from build123d import *

# Parameters (mm, degrees)
EXTRUDE_590_DEPTH   = 27.6
EXTRUDE_638_DEPTH   = 9.5
FILLET_1_R          = 3
HOLE_WIZARD_M5_1_D  = 5.3
CUT_EXTRUDE_1_DEPTH = 5
CUT_EXTRUDE_2_DEPTH = 0.1


with BuildPart() as part:
    # 草图1 → Extrude 590 (new body)
    with BuildSketch(Plane(origin=(0, 0, 0), x_dir=(1, 0, 0), z_dir=(0, 1, 0))):
        with BuildLine():
            Line((4.608867317, -165), (-4.608867317, -165))
            Line((-4.608867317, -165), (-5.444719551, -194.923972433))
            ThreePointArc((-5.444719551, -194.923972433), (0, -195), (5.444719551, -194.923972433))
            Line((5.444719551, -194.923972433), (4.608867317, -165))
        make_face()
    extrude(amount=EXTRUDE_590_DEPTH)

    # 草图1<3> → Extrude 638 (add)
    with BuildSketch(Plane(origin=(0, 0, 0), x_dir=(1, 0, 0), z_dir=(0, 1, 0))):
        with BuildLine():
            ThreePointArc((5.444719551, -194.923972433), (0, -195), (-5.444719551, -194.923972433))
            Line((-5.444719551, -194.923972433), (-5.584327745, -199.922023008))
            ThreePointArc((-5.584327745, -199.922023008), (0, -200), (5.584327745, -199.922023008))
            Line((5.584327745, -199.922023008), (5.444719551, -194.923972433))
        make_face()
    extrude(amount=EXTRUDE_638_DEPTH)

    # 圆角1
    fillet_1_edges = [part.edges().sort_by_distance(p)[0] for p in [
        (0, 0, 165),
        (-4.608867317, 13.8, 165),
        (4.608867317, 13.8, 165),
    ]]
    fillet(fillet_1_edges, radius=FILLET_1_R)

    # M5 间隙孔1 (through all)
    with Locations(Plane(origin=(0, 27.6, 0), x_dir=(1, 0, 0), z_dir=(0, 1, 0))):
        with Locations((0, -187), (0, -175)):
            Hole(HOLE_WIZARD_M5_1_D / 2)

    # 草图6 → 切除-拉伸1 (cut)
    with BuildSketch(Plane.XZ):
        Polygon((0, 179.792007234), (-4.15, 177.396003617), (-4.15, 172.603996383), (0, 170.207992766), (4.15, 172.603996383), (4.15, 177.396003617), align=None)
        Polygon((0, 191.792007234), (-4.15, 189.396003617), (-4.15, 184.603996383), (0, 182.207992766), (4.15, 184.603996383), (4.15, 189.396003617), align=None)
    extrude(amount=-CUT_EXTRUDE_1_DEPTH, mode=Mode.SUBTRACT)

    # 草图7 → 切除-拉伸2 (cut)
    with BuildSketch(Plane(origin=(0, 0, 0), x_dir=(-0.02792163872356911, 0, -0.9996101150403545), z_dir=(0.9996101150403545, 0, -0.02792163872356911))):
        Polygon((-170.936556358, 26.18974359), (-170.872754274, 26.18974359), (-170.872754274, 23.766666667), (-170.46890812, 23.766666667), (-170.46890812, 23.407692308), (-170.872754274, 23.407692308), (-170.872754274, 22.6), (-171.186856838, 22.6), (-171.186856838, 23.407692308), (-172.847113249, 23.407692308), align=None)
        Polygon((-171.186856838, 23.766666667), (-171.186856838, 25.286698718), (-172.230126069, 23.766666667), align=None, mode=Mode.SUBTRACT)
    extrude(amount=-CUT_EXTRUDE_2_DEPTH, mode=Mode.SUBTRACT)


solid = part.part
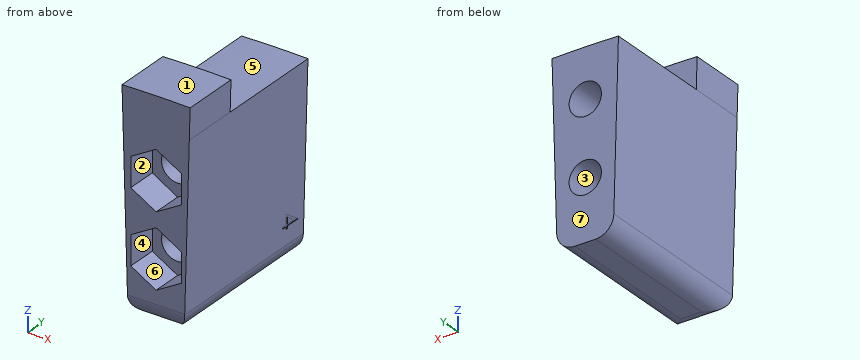
Check sheet for the modelled part. Datum: model origin and axes. Units: mm. Face numbers are marked on the shaded views. A direction names the side the tool comes from. Round coordinates to 2 decimals unless told otherwise and drop trailing zeros. Loops run counter-clockwise (first coordinate to the right, second up) from the corner with the lowest first, then second, coordinate; pieces in that order, holes last. Notation, with made-up numbers: M -4,-17 L 44,-17 A17 ccw 44,10 Z; hole C 62,67.5 d6. An arc over 180 degrees is marked long. One line per item, written item: value.
(1) Sectioned sample at A-A, the plane y = 3.5. Record the cut outline in (x, z).
Computed values:
outline: M -5.58,199.92 L -4.69,167.92 A3 ccw -1.69,165 L 1.69,165 A3 ccw 4.69,167.92 L 5.58,199.92 A200 ccw Z; hole M -4.15,172.6 L 0,170.21 L 4.15,172.6 L 4.15,177.4 L 0,179.79 L -4.15,177.4 Z; hole M -4.15,184.6 L 0,182.21 L 4.15,184.6 L 4.15,189.4 L 0,191.79 L -4.15,189.4 Z
(2) Release check for a two-part mould opening along Z. For the marked faces 4, 5, 6 and 7 record: +Z half, -Z half, draft (parallel to the pull), parting line (faces both ways), or undercut.
Computed values:
face 4: undercut
face 5: +Z half
face 6: undercut
face 7: draft
(3) Sectioned sample at D-D, the plane z = 179. Record the cut outline in (x, y).
Computed values:
outline: M -5,0 L -1.37,0 L -1.37,5 L 1.37,5 L 1.37,0 L 5,0 L 5,27.6 L -5,27.6 Z
(4) Access from +Z, -Z, +X, -X, +Y, -Y to the whole of each face (thin tool, end or side, straight path). Record for the marked faces 1, 2 and 3.
Computed values:
face 1: +Z, +Y, -Y
face 2: -Y
face 3: +Y, -Y
(5) Depth check by flat-ended pin: pin 1 Ø4 at (y, z) = (3.5, 174) entering from -X; pin 2 Ø6 at (y, z) = (12, 178) entering from -X; pin 3 Ø4 at (y, z) = (2, 175) entering from +X. Enter the tip coordinate at first touch or a pass-through.
Computed values:
pin 1: stops at x = -4.92
pin 2: stops at x = -5.06
pin 3: stops at x = 4.94
(6) Sectioned sample at B-B, the plane z = 175. Record the cut outline in (x, y), then the cut area to 3 significant figures.
Computed values:
outline: M -4.89,0 L -4.15,0 L -4.15,5 L -2.65,5 L -2.65,27.6 L -4.89,27.6 Z; M 2.65,5 L 4.15,5 L 4.15,0 L 4.89,0 L 4.89,27.6 L 2.65,27.6 Z
area: 109 mm^2
(7) Thickness scan on line 1 (Z direction, x = 0, y = 21.75); line 2 (Z direction, x = 0.75, y = 11.5); line 3 (Y direction, x = -3, z = 197). Record the ranges inside material, lowest first.
Computed values:
line 1: z = 165 to 172.35, 177.65 to 184.35, 189.65 to 195
line 2: z = 165 to 172.46, 177.54 to 184.46, 189.54 to 195
line 3: y = 0 to 9.5
(8) Sectioned sample at C-C, the plane y = 19. Record the cut outline in (x, z), then the cut area to 3 significant figures.
Computed values:
outline: M -5.44,194.92 L -4.69,167.92 A3 ccw -1.69,165 L 1.69,165 A3 ccw 4.69,167.92 L 5.44,194.92 A195 ccw Z; hole C 0,175 d5.3; hole C 0,187 d5.3
area: 254 mm^2
